Work out the finished part from the listing and answer in its coordinate system (mm). A direction names the side the tool comes from. Round coordinates to 2 decimals unless told otherwise and drop trailing zeros. Write each loop counter-clockwise with the first axis right and the second up, starting at its lowest first coordinate (ties: lowest second). Pieces come first, ordered by that corner, then holes. Notation, with made-up numbers: (20, 61) -> (37, 61) arc R11 ccw to (37, 67) -> close; hole circle Ø2 at (34.5, 16). An arc over 180 degrees is marked (long way). One line per item, written item: value.
```python
from build123d import *

# Parameters (mm, degrees)
SKIZZE2_W                       = 20
SKIZZE2_H                       = 20
AUFSATZ_LINEAR_AUSTRAGEN1_DEPTH = 25


with BuildPart() as part:
    # Skizze1 → Rotation1 (revolve)
    with BuildSketch(Plane.XY, mode=Mode.PRIVATE) as rotation1_sk:
        with BuildLine():
            Line((18.187375951, 0), (18.187375951, -18))
            Line((18.187375951, -18), (54.187375951, -18))
            ThreePointArc((54.187375951, -18), (57.015803076, -19.171572875), (58.187375951, -22))
            Line((58.187375951, -22), (58.187375951, -25))
            Line((58.187375951, -25), (68.187375951, -25))
            Line((68.187375951, -25), (68.187375951, -13))
            Line((68.187375951, -13), (72.187375951, -13))
            Line((72.187375951, -13), (72.187375951, -15))
            Line((72.187375951, -15), (108.187375951, -15))
            Line((108.187375951, -15), (108.187375951, -10))
            Line((108.187375951, -10), (124.187375951, -10))
            Line((124.187375951, -10), (126.187375951, -8))
            Line((126.187375951, -8), (126.187375951, 0))
            Line((126.187375951, 0), (18.187375951, 0))
        make_face()
    revolve(rotation1_sk.sketch.rotate(Axis((0, 0, 0), (1, 0, 0)), 270), axis=Axis((0, 0, 0), (1, 0, 0)))

    # Skizze2 → Aufsatz-Linear austragen1 (add)
    with BuildSketch(Plane.ZY.offset(-18.187375951)):
        Rectangle(SKIZZE2_W, SKIZZE2_H)
    extrude(amount=AUFSATZ_LINEAR_AUSTRAGEN1_DEPTH)


solid = part.part
```
(1) Flat-ended cylindrical pins translate along their axes: pin 1 Ø4 at (x, z) = (33.5, 8.5) entering from +Y; pin 2 Ø5 at (x, y) = (41.5, 13.5) entering from -Z; pin 3 Ø10 at (x, z) = (3, -3.5) entering from -Y. Find the tip coordinate at first contact, or state that the pin passes through.
Reported:
pin 1: stops at y = 16.79
pin 2: stops at z = -14.25
pin 3: stops at y = -10
(2) Find section A-A on y = 0. Give the vertices of the cut face in (x, z), plus the area to 3 significant figures.
Reported:
outline: (-6.81, -10) -> (18.19, -10) -> (18.19, -18) -> (54.19, -18) arc R4 cw to (58.19, -22) -> (58.19, -25) -> (68.19, -25) -> (68.19, -13) -> (72.19, -13) -> (72.19, -15) -> (108.19, -15) -> (108.19, -10) -> (124.19, -10) -> (126.19, -8) -> (126.19, 8) -> (124.19, 10) -> (108.19, 10) -> (108.19, 15) -> (72.19, 15) -> (72.19, 13) -> (68.19, 13) -> (68.19, 25) -> (58.19, 25) -> (58.19, 22) arc R4 cw to (54.19, 18) -> (18.19, 18) -> (18.19, 10) -> (-6.81, 10) -> close
area: 3,990 mm2
(3) Consider probe 1 along Y at (x, z) = (11, 0.5); probe 2 along X at (y, z) = (-8, -21); probe 3 along X at (y, z) = (-11, -2.5). Determine where each line is inside the solid, lowest interval first.
Reported:
probe 1: y = -10 to 10
probe 2: x = 58.19 to 68.19
probe 3: x = 18.19 to 108.19
(4) Find section D-D on x = 7. Give the vertices of the cut face in (y, z).
Reported:
outline: (-10, -10) -> (10, -10) -> (10, 10) -> (-10, 10) -> close
(5) A tool of negligible diameter and unlimited length cuts with its end or side. For faces 1 (the face through (6, 0, 10)), 2 (the face through (6, 10, 0)), 3 (the face through (58.187, 22.1, -1.7)), 4 (the face through (6, -10, 0)), 5 (the face through (6, 0, -10)), from which of +Z, -Z, +X, -X, +Y, -Y can it reach the whole face along a straight path? Write none if from no direction.
Reported:
face 1: +Z, -X, +Y, -Y
face 2: +Z, -Z, -X, +Y
face 3: -X
face 4: +Z, -Z, -X, -Y
face 5: -Z, -X, +Y, -Y
(6) Find section C-C on x = 24. Give the vertices of the cut face in (y, z).
Reported:
outline: circle Ø36 at (0, 0)
(7) For a pull along X with two mould halves and no side action, classify faces 6 (the face through (72.187, -13.4, 0.1)), 7 (the face through (108.187, 3, 10)), 8 (the face through (70.215, 7.91, -10.316)), 9 (the face through (63.257, -7.509, 23.846)) as pulls with the +X half, pulls with the -X half, needs draft (parallel to the pull), parting line crosses it, or undercut.
Reported:
face 6: undercut
face 7: pulls with the +X half
face 8: undercut
face 9: needs draft
